Verification items for this drawing (mm, ordinates from the low corner). Round coordinates to 2 decimals unless told otherwise and drop trailing zeros. Loops run counter-clockwise (first coordinate to the right, second up) from the corner with the lowest first, then second, coordinate; pieces in that order, holes last. Notation, with made-up numbers: M 12,11.25 L 28,11.25 A19 cw 28,35.25 Z; hole C 17.25,59 d7. An arc over 180 degrees is marked long. Answer as CSV lines item,"result".
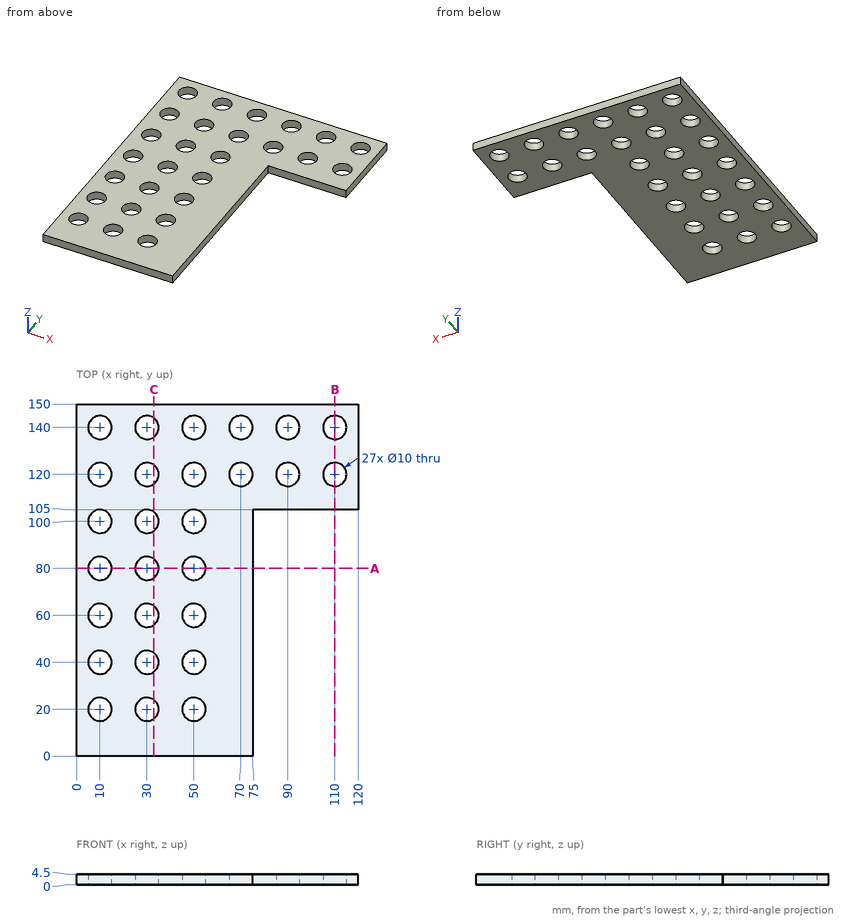
1) Section check B-B (x = 110). Record the cut outline in (y, z), plus the area to 4 significant figures.
Here are the results:
outline,"M 105,0 L 115,0 L 115,4.5 L 105,4.5 Z; M 125,0 L 135,0 L 135,4.5 L 125,4.5 Z; M 145,0 L 150,0 L 150,4.5 L 145,4.5 Z"
area,"112.5 mm^2"
2) Section check A-A (y = 80). Record the cut outline in (x, z).
Here are the results:
outline,"M 0,0 L 5,0 L 5,4.5 L 0,4.5 Z; M 15,0 L 25,0 L 25,4.5 L 15,4.5 Z; M 35,0 L 45,0 L 45,4.5 L 35,4.5 Z; M 55,0 L 75,0 L 75,4.5 L 55,4.5 Z"
3) Section check C-C (x = 33). State how many separate pieces and enclosed holes the cut face has, plus the area to 3 significant figures.
Here are the results:
separate pieces,"8"
enclosed holes,"0"
area,"423 mm^2"
4) Material ranges on probe 1 along Y at (x, z) = (106, 0.85); probe 2 along X at (y, z) = (64, 1.05); probe 3 along X at (y, z) = (103.5, 4.1), recorded low to high.
Here are the results:
probe 1,"y = 105 to 117, 123 to 137, 143 to 150"
probe 2,"x = 0 to 7, 13 to 27, 33 to 47, 53 to 75"
probe 3,"x = 0 to 6.43, 13.57 to 26.43, 33.57 to 46.43, 53.57 to 75"
5) Go/stop test with flat-tipped pins: pin 1 (11.5 mm diameter, centred on x = 110, y = 120, fed in from +Z); pin 2 (6 mm diameter, centred on x = 50, y = 120, fed in from -Z); pin 3 (1.5 mm diameter, centred on x = 88, z = 2, fed in from -Y); pin 4 (1.5 mm diameter, centred on y = 89, z = 2.5, fed in from +X). Record where each tip stops, or that it passes through.
Here are the results:
pin 1,"stops at z = 4.5"
pin 2,"passes through"
pin 3,"stops at y = 105"
pin 4,"stops at x = 75"
